Part print with two shaded views. Sizes in mm from the minimum x, y, z corner. A direction names the side the tool comes from. Give positions to 0.01 mm unless a question says otherwise; leave off trailing zeros. Write each loop counter-clockwise with the first axis right and the second up, starting at its lowest first coordinate (ties: lowest second). Pieces come first, ordered by that corner, then holes. Notation, with made-up numbers: (-28.5, 75.25) - (-6.5, 75.25) arc R9 ccw to (-6.5, 83.25) - close; hole circle Ø8 at (86.25, -28.75). An arc over 180 degrees is marked (long way). Answer as a JSON object with one key per item and string values.
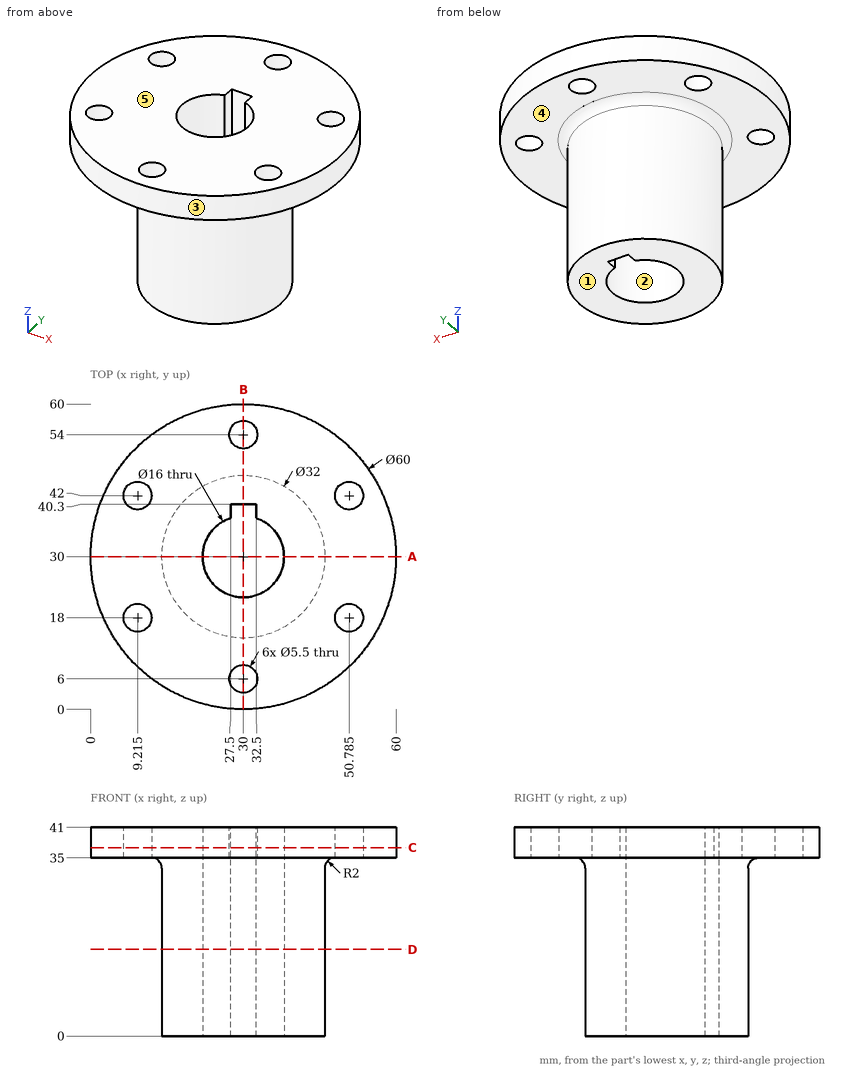
(1) Saw through at C-C, the plane z = 37. State how many separate pieces and enclosed holes the cut face has, and give its area (3 significant figures).
Answer key:
{"separate pieces": "1", "enclosed holes": "7", "area": "2,470 mm²"}
(2) Flat gauge pins, fed straight in: P1, Ø2, axis at y = 39, z = 28, coming from the +X side; P2, Ø2, axis at y = 39, z = 14, coming from the -X side; P3, Ø4, axis at x = 18, z = 28, coming from the -Y side; P4, Ø5, axis at x = 30, y = 54, coming from the +Z side. Where does each tip first touch, or does it go through?
Answer key:
{"P1": "stops at x = 43.86", "P2": "stops at x = 16.14", "P3": "stops at y = 17.51", "P4": "passes through"}
(3) Probe L1, parallel to Y at x = 30, z = 36; L2, parallel to Y at x = 49, z = 38 (1 decimal); L3, parallel to Y at x = 30, z = 33. List the from-to ranges inside material, lowest first. Write a range as [from, to].
Answer key:
{"L1": "y = [0, 3.25], [8.75, 22], [40.3, 51.25], [56.75, 60]", "L2": "y = [6.8, 15.9], [20.1, 39.9], [44.1, 53.2]", "L3": "y = [14, 22], [40.3, 46]"}
(4) Saw through at B-B, the plane x = 30. Give the cut face in (y, z).
Answer key:
{"outline": "(0, 35) - (3.25, 35) - (3.25, 41) - (0, 41) - close; (8.75, 35) - (12, 35) arc R2 cw to (14, 33) - (14, 0) - (22, 0) - (22, 41) - (8.75, 41) - close; (40.3, 0) - (46, 0) - (46, 33) arc R2 cw to (48, 35) - (51.25, 35) - (51.25, 41) - (40.3, 41) - close; (56.75, 35) - (60, 35) - (60, 41) - (56.75, 41) - close"}
(5) 3-axis set-ups, long thin cutter, end or side, ignore diameter. For the marked faces 4 and 5: which of +Z, -Z, +X, -X, +Y, -Y reach the whole face in a straight line?
Answer key:
{"face 4": "-Z", "face 5": "+Z, +X, -X, +Y, -Y"}
(6) Saw through at D-D, the plane z = 17. Give the cut face in (x, y), and give its area (3 significant figures).
Answer key:
{"outline": "circle Ø32 at (30, 30); hole (27.5, 37.6) arc R8 ccw (long way) to (32.5, 37.6) - (32.5, 40.3) - (27.5, 40.3) - close", "area": "591 mm²"}
(7) Saw through at A-A, the plane y = 30. Give the cut face in (x, z).
Answer key:
{"outline": "(0, 35) - (12, 35) arc R2 cw to (14, 33) - (14, 0) - (22, 0) - (22, 41) - (0, 41) - close; (38, 0) - (46, 0) - (46, 33) arc R2 cw to (48, 35) - (60, 35) - (60, 41) - (38, 41) - close"}
(8) Pull direction X, two halves, no side cores. Call the marked faces 1, 2 and 3: pulls with the +X half, pulls with the -X half, needs draft (parallel to the pull), parting line crosses it, or undercut.
Answer key:
{"face 1": "needs draft", "face 2": "undercut", "face 3": "parting line crosses it"}
